from build123d import *

# Parameters (mm, degrees)
SKETCH1_R           = 6
SKETCH1_R_2         = 2
BOSS_EXTRUDE1_DEPTH = 4
FILLET1_R           = 0.5
SKETCH2_R           = 4.9
SKETCH2_R_2         = 3.4
CUT_EXTRUDE1_DEPTH  = 0.5
SKETCH3_R           = 4.9
SKETCH3_R_2         = 3.4
CUT_EXTRUDE2_DEPTH  = 0.5


with BuildPart() as part:
    # Sketch1 → Boss-Extrude1 (new body)
    with BuildSketch(Plane(origin=(0, 0, 0), x_dir=(0, 0, -1), z_dir=(1, 0, 0))):
        Circle(SKETCH1_R)
        Circle(SKETCH1_R_2, mode=Mode.SUBTRACT)
    extrude(amount=BOSS_EXTRUDE1_DEPTH)

    # Fillet1
    fillet1_edges = [part.edges().sort_by_distance(p)[0] for p in [
        (0, 0, 6),
        (4, 0, 6),
    ]]
    fillet(fillet1_edges, radius=FILLET1_R)

    # Sketch2 → Cut-Extrude1 (cut)
    with BuildSketch(Plane(origin=(4, 0, 0), x_dir=(0, 0, -1), z_dir=(1, 0, 0))):
        Circle(SKETCH2_R)
        Circle(SKETCH2_R_2, mode=Mode.SUBTRACT)
    extrude(amount=-CUT_EXTRUDE1_DEPTH, mode=Mode.SUBTRACT)

    # Sketch3 → Cut-Extrude2 (cut)
    with BuildSketch(Plane.ZY):
        Circle(SKETCH3_R)
        Circle(SKETCH3_R_2, mode=Mode.SUBTRACT)
    extrude(amount=-CUT_EXTRUDE2_DEPTH, mode=Mode.SUBTRACT)


solid = part.part
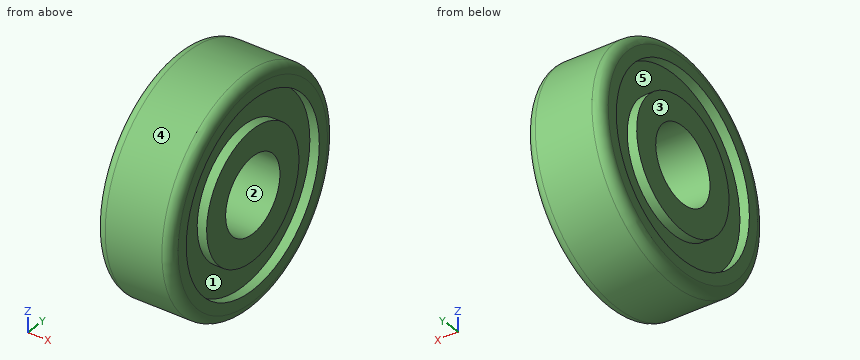
Here's how the part is built. I have some questions about the finished solid (model axes, mm). Face numbers are marked on the shaded views. A direction names the side the tool comes from. Coordinates: 2 decimals unless noted, no trailing zeros. Order: outer loops, then holes, each group sorted by start corner. A loop starts at its lowest first (then second) coordinate and runs counter-clockwise, first axis right, second up. Notation, with made-up numbers: (68.25, 29.25) -> (119.25, 29.25) arc R25 ccw to (119.25, 64.25) -> close; hole circle Ø11 at (25.5, 1). An arc over 180 degrees is marked (long way). Answer in a Markdown table with one row per item.
(1) Will these pins go through, and if not, where does the flat tip stop? pin 1 Ø1.5 at (x, z) = (3, -1.5) entering from -Y; pin 2 Ø1 at (y, z) = (4, 0) entering from -X; pin 3 Ø3 at (y, z) = (0, 0) entering from +X.
Answer key:
| item | result |
|---|---|
| pin 1 | y = -5.95 |
| pin 2 | x = 0.5 |
| pin 3 | through |
(2) Thinking about a two-plate mould opening in Z: for the marked faces 3, 4 and 5, which applies, +Z half, -Z half, draft (parallel to the pull), parting line (faces both ways), or undercut?
Answer key:
| item | result |
|---|---|
| face 3 | draft |
| face 4 | parting line |
| face 5 | undercut |
(3) I want a section at A-A on y = 0. List the corners of the cut face in (x, z) for me.
Answer key:
| item | result |
|---|---|
| outline | (0, -5.5) arc R0.5 ccw to (0.5, -6) -> (3.5, -6) arc R0.5 ccw to (4, -5.5) -> (4, -4.9) -> (3.5, -4.9) -> (3.5, -3.4) -> (4, -3.4) -> (4, -2) -> (0, -2) -> (0, -3.4) -> (0.5, -3.4) -> (0.5, -4.9) -> (0, -4.9) -> close; (0, 2) -> (4, 2) -> (4, 3.4) -> (3.5, 3.4) -> (3.5, 4.9) -> (4, 4.9) -> (4, 5.5) arc R0.5 ccw to (3.5, 6) -> (0.5, 6) arc R0.5 ccw to (0, 5.5) -> (0, 4.9) -> (0.5, 4.9) -> (0.5, 3.4) -> (0, 3.4) -> close |
(4) Please list where these lines run through material, in increasing order: probe 1 along Y at (x, z) = (0.3, -2.25); probe 2 along Y at (x, z) = (3.7, 0); probe 3 along Z at (x, y) = (3.55, -1.5).
Answer key:
| item | result |
|---|---|
| probe 1 | -5.52 to -4.35, -2.55 to 2.55, 4.35 to 5.52 |
| probe 2 | -5.96 to -4.9, -3.4 to -2, 2 to 3.4, 4.9 to 5.96 |
| probe 3 | -5.81 to -4.66, -3.05 to -1.32, 1.32 to 3.05, 4.66 to 5.81 |
(5) I want a section at D-D on x = 2.1. List the corners of the cut face in (y, z) for me.
Answer key:
| item | result |
|---|---|
| outline | circle Ø12 at (0, 0); hole circle Ø4 at (0, 0) |
(6) I want a section at C-C on x = 3.7. List the corners of the cut face in (y, z) for me, then the cut area to 4 significant figures.
Answer key:
| item | result |
|---|---|
| outline | circle Ø11.92 at (0, 0); circle Ø6.8 at (0, 0); hole circle Ø9.8 at (0, 0); hole circle Ø4 at (0, 0) |
| area | 59.85 mm^2 |
(7) On a 3-axis mill with a long thin cutter (end or side, diameter ignored), from which of +Z, -Z, +X, -X, +Y, -Y can I reach the whole of each face in a straight line? I mean the marked faces 1 and 2. Say none if no direction works.
Answer key:
| item | result |
|---|---|
| face 1 | +X |
| face 2 | +X, -X |
